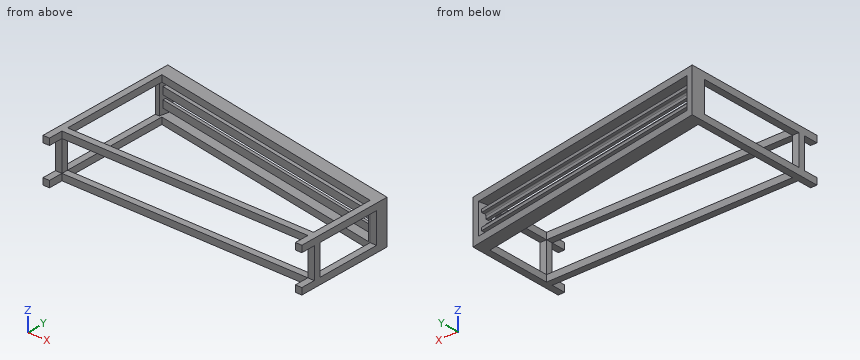
from build123d import *

# Parameters (mm, degrees)
RESSALTO_EXTRUS_O1_DEPTH = 300
ESBO_O2_W                = 1710
ESBO_O2_H                = 100
CORTE_EXTRUS_O1_DEPTH    = 300
CORTE_EXTRUS_O2_START    = -1800
ESBO_O3_W                = 210
ESBO_O3_H                = 454.157753787
ESBO_O3_H_2              = 100
CORTE_EXTRUS_O2_DEPTH    = 1800
ESBO_O4_W                = 1710
ESBO_O4_H                = 210
CORTE_EXTRUS_O3_DEPTH    = 45
ESBO_O5_W                = 210
ESBO_O5_H                = 301.519137011
CORTE_EXTRUS_O4_DEPTH    = 45
ESBO_O6_W                = 1737.767901394
ESBO_O6_H                = 210
CORTE_EXTRUS_O5_DEPTH    = 150
RESSALTO_EXTRUS_O2_DEPTH = 1737.767901394
FILETE1_R                = 10


with BuildPart() as part:
    # Esboço1 → Ressalto-extrusão1 (new body)
    with BuildSketch(Plane.XY):
        Polygon((0, 1000), (0, 0), (1800, 0), (1800, 682.611434725), align=None)
    extrude(amount=RESSALTO_EXTRUS_O1_DEPTH)

    # Esboço2 → Corte-extrusão1 (cut)
    with BuildSketch(Plane.XY.offset(300)):
        with Locations((900, 50)):
            Rectangle(ESBO_O2_W, ESBO_O2_H)
        Polygon((45, 900.676890798), (45, 145), (1755, 145), (1755, 599.157753787), align=None)
    extrude(amount=-CORTE_EXTRUS_O1_DEPTH, mode=Mode.SUBTRACT)

    # Esboço3 → Corte-extrusão2 (cut)
    with BuildSketch(Plane(origin=(1800, 0, 0), x_dir=(0, 0, -1), z_dir=(1, 0, 0)).offset(CORTE_EXTRUS_O2_START)):
        with Locations((-150, 372.078876894)):
            Rectangle(ESBO_O3_W, ESBO_O3_H)
        with Locations((-150, 50)):
            Rectangle(ESBO_O3_W, ESBO_O3_H_2)
    extrude(amount=CORTE_EXTRUS_O2_DEPTH, mode=Mode.SUBTRACT)

    # Esboço4 → Corte-extrusão3 (cut)
    with BuildSketch(Plane(origin=(0, 145, 0), x_dir=(1, 0, 0), z_dir=(0, 1, 0))):
        with Locations((900, -150)):
            Rectangle(ESBO_O4_W, ESBO_O4_H)
    extrude(amount=-CORTE_EXTRUS_O3_DEPTH, mode=Mode.SUBTRACT)

    # Esboço5 → Corte-extrusão4 (cut)
    with BuildSketch(Plane(origin=(45, 0, 0), x_dir=(0, 0, -1), z_dir=(1, 0, 0))):
        with Locations((-150, 749.917322293)):
            Rectangle(ESBO_O5_W, ESBO_O5_H)
    extrude(amount=-CORTE_EXTRUS_O4_DEPTH, mode=Mode.SUBTRACT)

    # Esboço6 → Corte-extrusão5 (cut)
    with BuildSketch(Plane(origin=(171.010071663, 969.846310393, 0), x_dir=(0.9848077530122075, -0.17364817766693394, 0), z_dir=(0.17364817766693397, 0.9848077530122076, 0))):
        with Locations((740.23577303, -150)):
            Rectangle(ESBO_O6_W, ESBO_O6_H)
    extrude(amount=-CORTE_EXTRUS_O5_DEPTH, mode=Mode.SUBTRACT)

    # Esboço8 → Ressalto-extrusão2 (add)
    with BuildSketch(Plane(origin=(-126.693722777, 22.339521612, 0), x_dir=(0, 0, -1), z_dir=(0.9848077530122076, -0.173648177666934, 0))):
        Polygon((-215, 964.807753012), (-215, 914.807753012), (-165, 914.807753012), (-165, 934.807753012), (-195, 934.807753012), (-195, 964.807753012), align=None)
        Polygon((-135, 914.807753012), (-85, 914.807753012), (-85, 964.807753012), (-105, 964.807753012), (-105, 934.807753012), (-135, 934.807753012), align=None)
    extrude(amount=RESSALTO_EXTRUS_O2_DEPTH)

    # Filete1
    filete1_edges = [part.edges().sort_by_distance(p)[0] for p in [
        (891.317591116, 792.065329712, 195),
        (891.317591116, 792.065329712, 105),
    ]]
    fillet(filete1_edges, radius=FILETE1_R)


solid = part.part
Geometry: final body of the model. Coordinates: model frame, mm. Round coordinates to 2 decimals unless told otherwise and drop trailing zeros. Order: outer loops, then holes, each group sorted by start corner. A loop starts at its lowest first (then second) coordinate and runs counter-clockwise, first axis right, second up. Notation, with made-up numbers: (60, -16) -> (99, -16) arc R22 ccw to (99, -4) -> close; hole circle Ø4 at (75, 3.25). An arc over 180 degrees is marked (long way). Put each result on its own line as item: value. Start each with the question number.
Q1. First-contact query: pin 1 (10 mm diameter, centred on x = 742, z = 252, fed in from +Y). Flat tip, straight axial feed; report the tip coordinate or a pass-through.
Q2. Line query: probe 1 along Z at (x, y) = (1101, 747); probe 2 along X at (y, z) = (545, 270); probe 3 along Z at (x, y) = (1103.5, 109). Output: solid intervals per line, ascending.
Q3. Section B-B on x = 738. Give the number of separate pieces and of enclosed holes in the cut face, and give its area (3 significant figures).
Q4. Section A-A on y = 256.5. Return the cut outline in (x, z), and give its area (3 significant figures).
Ans:
1. pin 1: stops at y = 869.87
2. probe 1: z = 0 to 45, 85 to 135, 165 to 215, 255 to 300
2. probe 2: x = 0 to 45, 1755 to 1800
2. probe 3: z = 0 to 45, 255 to 300
3. separate pieces: 6
3. enclosed holes: 0
3. area: 15,600 mm2
4. outline: (0, 0) -> (45, 0) -> (45, 45) -> (0, 45) -> close; (0, 255) -> (45, 255) -> (45, 300) -> (0, 300) -> close; (1755, 0) -> (1800, 0) -> (1800, 45) -> (1755, 45) -> close; (1755, 255) -> (1800, 255) -> (1800, 300) -> (1755, 300) -> close
4. area: 8,100 mm2
